For this review, take the finished solid that the model builds, in its own axes (mm). Face numbers are marked on the shaded views. A direction names the side the tool comes from. Coordinates: 2 decimals unless noted, no trailing zeros. Order: outer loops, then holes, each group sorted by start corner. A loop starts at its lowest first (then second) coordinate and runs counter-clockwise, first axis right, second up. Notation, with made-up numbers: M 87,-17 L 102,-17 A25 ccw 102,22 Z; hole C 1,-24 d11. An arc over 180 degrees is marked long. Use one line per item in the form item = value. Start each with the question number.
```python
from build123d import *

# Parameters (mm, degrees)
BASE_FLANGE1_DEPTH = 80
SKETCH6_R          = 1
SKETCH6_W          = 24
SKETCH6_H          = 13
CUT_EXTRUDE1_DEPTH = 161.141019336
SKETCH7_W          = 20
SKETCH7_H          = 40
CUT_EXTRUDE2_DEPTH = 10


# Sheet-metal steps are written as plain solids
with BuildPart() as part:
    # Sketch1 → Base-Flange1 (new body)
    with BuildSketch(Plane(origin=(0, 0, 0), x_dir=(1, 0, 0), z_dir=(0, 0, -1))):
        with BuildLine():
            Line((50.5, -60.295787408), (50.5, -83.295787408))
            ThreePointArc((50.5, -83.295787408), (49.914213562, -84.710000971), (48.5, -85.295787408))
            Line((48.5, -85.295787408), (24.5, -85.295787408))
            ThreePointArc((24.5, -85.295787408), (23.085786438, -84.710000971), (22.5, -83.295787408))
            Line((22.5, -83.295787408), (22.5, -65.295787408))
            ThreePointArc((22.5, -65.295787408), (21.035533906, -61.760253502), (17.5, -60.295787408))
            Line((17.5, -60.295787408), (-17.5, -60.295787408))
            ThreePointArc((-17.5, -60.295787408), (-21.035533906, -61.760253502), (-22.5, -65.295787408))
            Line((-22.5, -65.295787408), (-22.5, -83.295787408))
            ThreePointArc((-22.5, -83.295787408), (-23.085786438, -84.710000971), (-24.5, -85.295787408))
            Line((-24.5, -85.295787408), (-48.5, -85.295787408))
            ThreePointArc((-48.5, -85.295787408), (-49.914213562, -84.710000971), (-50.5, -83.295787408))
            Line((-50.5, -83.295787408), (-50.5, -60.295787408))
            Line((-50.5, -60.295787408), (-53.5, -60.295787408))
            Line((-53.5, -60.295787408), (-53.5, -83.295787408))
            ThreePointArc((-53.5, -83.295787408), (-52.035533906, -86.831321314), (-48.5, -88.295787408))
            Line((-48.5, -88.295787408), (-24.5, -88.295787408))
            ThreePointArc((-24.5, -88.295787408), (-20.964466094, -86.831321314), (-19.5, -83.295787408))
            Line((-19.5, -83.295787408), (-19.5, -65.295787408))
            ThreePointArc((-19.5, -65.295787408), (-18.914213562, -63.881573846), (-17.5, -63.295787408))
            Line((-17.5, -63.295787408), (17.5, -63.295787408))
            ThreePointArc((17.5, -63.295787408), (18.914213562, -63.881573846), (19.5, -65.295787408))
            Line((19.5, -65.295787408), (19.5, -83.295787408))
            ThreePointArc((19.5, -83.295787408), (20.964466094, -86.831321314), (24.5, -88.295787408))
            Line((24.5, -88.295787408), (48.5, -88.295787408))
            ThreePointArc((48.5, -88.295787408), (52.035533906, -86.831321314), (53.5, -83.295787408))
            Line((53.5, -83.295787408), (53.5, -60.295787408))
            Line((53.5, -60.295787408), (50.5, -60.295787408))
        make_face()
    extrude(amount=BASE_FLANGE1_DEPTH)

    # Sketch6 → Cut-Extrude1 (cut, through all)
    with BuildSketch(Plane.ZY.offset(53.5)):
        with Locations(Location((-38.674720748, 71.795787408, 0), (0, 0, 90))):
            Circle(SKETCH6_R)
        with Locations(Location((-10.874720748, 71.795787408, 0), (0, 0, 90))):
            Circle(SKETCH6_R)
        with Locations((-24.774720748, 71.795787408)):
            Rectangle(SKETCH6_W, SKETCH6_H)
    extrude(amount=-CUT_EXTRUDE1_DEPTH, mode=Mode.SUBTRACT)

    # Sketch7 → Cut-Extrude2 (cut)
    with BuildSketch(Plane(origin=(0, 88.295787408, 0), x_dir=(1, 0, 0), z_dir=(0, 1, 0))):
        with Locations((-36.5, 22)):
            Rectangle(SKETCH7_W, SKETCH7_H)
        with Locations((36.5, 22)):
            Rectangle(SKETCH7_W, SKETCH7_H)
    extrude(amount=-CUT_EXTRUDE2_DEPTH, mode=Mode.SUBTRACT)


solid = part.part
```
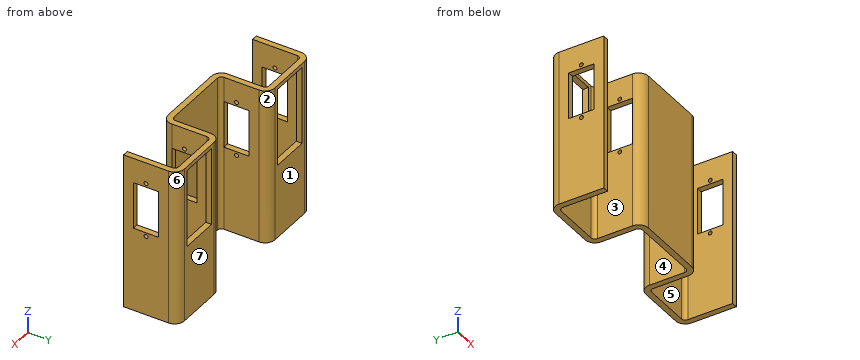
1. Consider section A-A, the plane y = 76.25. Give the number of separate pieces and of enclosed holes in the cut face, plus the area to 3 significant figures.
2. Consider section B-B, the plane x = 28. Write out the cut boundary in (y, z).
3. For pin 1 Ø0.9 at (y, z) = (86.5, -17) entering from -X; pin 2 Ø3.5 at (x, z) = (-52, -23.5) entering from +Y; pin 3 Ø2 at (x, z) = (12, -36) entering from +Y, all flat-tipped, find the tip position at first contact; note any pin that passes through.
4. The part is to be moulded in two halves that separate along X. For the marked faces 4, 5, 6 and 7, say which applies: pulls with the +X half, pulls with the -X half, needs draft (parallel to the pull), parting line crosses it, or undercut.
5. Tool access review of the marked faces 1, 2 and 3: name each direction out of +Z, -Z, +X, -X, +Y, -Y from which nothing blocks a thin tool from reaching the whole face with its end or side.
6. Consider section C-C, the plane z = -60.5. Write out the cut boundary in (x, y), plus the area to 3 significant figures.
7. To check wall thickness, follow line 1 (X direction, y = 67.25, z = -65.5); line 2 (X direction, y = 87, z = -41.5); line 3 (Y direction, x = -46, z = -66.5). State the ranges of each line that lie inside material, in increasing order.
Answers follow:
q1.separate_pieces = 8
q1.enclosed_holes = 0
q1.area = 672 mm²
q2.outline = M 85.3,-80 L 88.3,-80 L 88.3,-42 L 85.3,-42 Z; M 85.3,-2 L 88.3,-2 L 88.3,0 L 85.3,0 Z
q3.pin_1 = -52.67
q3.pin_2 = 87.98
q3.pin_3 = 63.3
q4.face_4 = undercut
q4.face_5 = undercut
q4.face_6 = pulls with the +X half
q4.face_7 = needs draft
q5.face_1 = +Z, -Z, +X, -X, +Y
q5.face_2 = +Z, -Z, +Y
q5.face_3 = +Z, -Z, -Y
q6.outline = M -53.5,60.3 L -50.5,60.3 L -50.5,83.3 A2 cw -48.5,85.3 L -24.5,85.3 A2 cw -22.5,83.3 L -22.5,65.3 A5 ccw -17.5,60.3 L 17.5,60.3 A5 ccw 22.5,65.3 L 22.5,83.3 A2 cw 24.5,85.3 L 48.5,85.3 A2 cw 50.5,83.3 L 50.5,60.3 L 53.5,60.3 L 53.5,83.3 A5 ccw 48.5,88.3 L 24.5,88.3 A5 ccw 19.5,83.3 L 19.5,65.3 A2 cw 17.5,63.3 L -17.5,63.3 A2 cw -19.5,65.3 L -19.5,83.3 A5 ccw -24.5,88.3 L -48.5,88.3 A5 ccw -53.5,83.3 Z
q6.area = 594 mm²
q7.line_1 = -53.5 to -50.5, -22.5 to -19.5, 19.5 to 22.5, 50.5 to 53.5
q7.line_2 = -51.86 to -46.5, -26.5 to -21.14, 21.14 to 26.5, 46.5 to 51.86
q7.line_3 = 85.3 to 88.3
